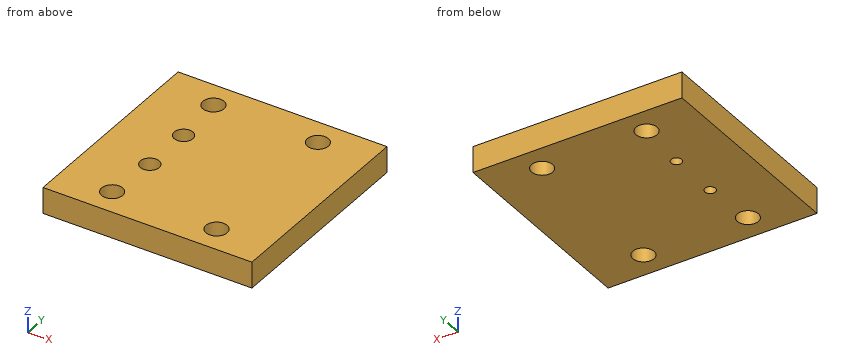
from build123d import *

# Parameters (mm, degrees)
F0_W     = 80
F0_H     = 80
F0_R     = 4.05
F0_R_2   = 2.025
F1_DEPTH = 10
F2_R     = 3.6
F3_DEPTH = 5


with BuildPart() as f1:
    # F0 (on Top) → F1 (new body)
    with BuildSketch(Plane.XY):
        with Locations((40, -40)):
            Rectangle(F0_W, F0_H)
        with Locations((20, -70)):
            Circle(F0_R, mode=Mode.SUBTRACT)
        with Locations((21.5, -50)):
            Circle(F0_R_2, mode=Mode.SUBTRACT)
        with Locations((60, -70)):
            Circle(F0_R, mode=Mode.SUBTRACT)
        with Locations((21.5, -30)):
            Circle(F0_R_2, mode=Mode.SUBTRACT)
        with Locations((20, -10)):
            Circle(F0_R, mode=Mode.SUBTRACT)
        with Locations((60, -10)):
            Circle(F0_R, mode=Mode.SUBTRACT)
    extrude(amount=F1_DEPTH)

    # F2 (on face) → F3 (cut)
    with BuildSketch(Plane.XY.offset(10)):
        with Locations((21.5, -30)):
            Circle(F2_R)
        with Locations((21.5, -50)):
            Circle(F2_R)
    extrude(amount=-F3_DEPTH, mode=Mode.SUBTRACT)


solid = f1.part
For this review, take the finished solid that the model builds, in its own axes (mm). Give positions to 0.01 mm unless a question says otherwise; leave off trailing zeros. Order: outer loops, then holes, each group sorted by start corner. A loop starts at its lowest first (then second) coordinate and runs counter-clockwise, first axis right, second up. Notation, with made-up numbers: (79, 34) -> (92, 34) arc R34 cw to (92, 71) -> close; hole circle Ø4 at (-36.75, 30.25). An arc over 180 degrees is marked (long way). Write item = value, one per line.
1) To check wall thickness, follow L1, parallel to Y at x = 60, z = 5.5; L2, parallel to X at y = -12, z = 5.75; L3, parallel to Y at x = 21.5, z = 6.45. State the ranges of each line that lie inside material, in increasing order. Write a range as from..to.
Findings:
L1 = -80..-74.05, -65.95..-14.05, -5.95..0
L2 = 0..16.48, 23.52..56.48, 63.52..80
L3 = -80..-73.76, -66.24..-53.6, -46.4..-33.6, -26.4..-13.76, -6.24..0
2) We need section B-B, the plane z = 6.5. Give the boundary of the cut face in (x, y), and give its area (3 significant figures).
Findings:
outline = (0, -80) -> (80, -80) -> (80, 0) -> (0, 0) -> close; hole circle Ø8.1 at (20, -70); hole circle Ø8.1 at (20, -10); hole circle Ø7.2 at (21.5, -50); hole circle Ø7.2 at (21.5, -30); hole circle Ø8.1 at (60, -70); hole circle Ø8.1 at (60, -10)
area = 6,110 mm^2
3) We need section D-D, the plane x = 57.5. Give the boundary of the cut face in (y, z).
Findings:
outline = (-80, 0) -> (-73.19, 0) -> (-73.19, 10) -> (-80, 10) -> close; (-66.81, 0) -> (-13.19, 0) -> (-13.19, 10) -> (-66.81, 10) -> close; (-6.81, 0) -> (0, 0) -> (0, 10) -> (-6.81, 10) -> close
4) We need section A-A, the plane y = -10. Give the boundary of the cut face in (x, z).
Findings:
outline = (0, 0) -> (15.95, 0) -> (15.95, 10) -> (0, 10) -> close; (24.05, 0) -> (55.95, 0) -> (55.95, 10) -> (24.05, 10) -> close; (64.05, 0) -> (80, 0) -> (80, 10) -> (64.05, 10) -> close
5) Insertion check: pin 1 (4.5 mm diameter, centred on x = 21.5, y = -30, fed in from +Z); pin 2 (2.5 mm diameter, centred on x = 21.5, y = -50, fed in from -Z). Each pin has a flat end and moves straight along its axis. Give the tip position at first contact, or say it passes through.
Findings:
pin_1 = 5
pin_2 = through
6) We need section C-C, the plane y = -30. Give the boundary of the cut face in (x, z) (3 decimals), and give its area (3 significant figures).
Findings:
outline = (0, 0) -> (19.475, 0) -> (19.475, 5) -> (17.9, 5) -> (17.9, 10) -> (0, 10) -> close; (23.525, 0) -> (80, 0) -> (80, 10) -> (25.1, 10) -> (25.1, 5) -> (23.525, 5) -> close
area = 744 mm^2
